For this review, use the dimensioned drawing (mm, ordinates from the lowest corner) and the shaded views. A direction names the side the tool comes from. Give positions to 0.01 mm unless a question says otherwise; leave off trailing zeros. Write each loop counter-clockwise with the first axis right and the second up, starting at its lowest first coordinate (ties: lowest second). Pieces come first, ordered by that corner, then holes. Notation, with made-up numbers: (8.25, 88) -> (61.25, 88) arc R28 cw to (61.25, 109) -> close; hole circle Ø1 at (3, -9.5). An arc over 180 degrees is marked (long way). Return JSON: item names as keys, results as strings.
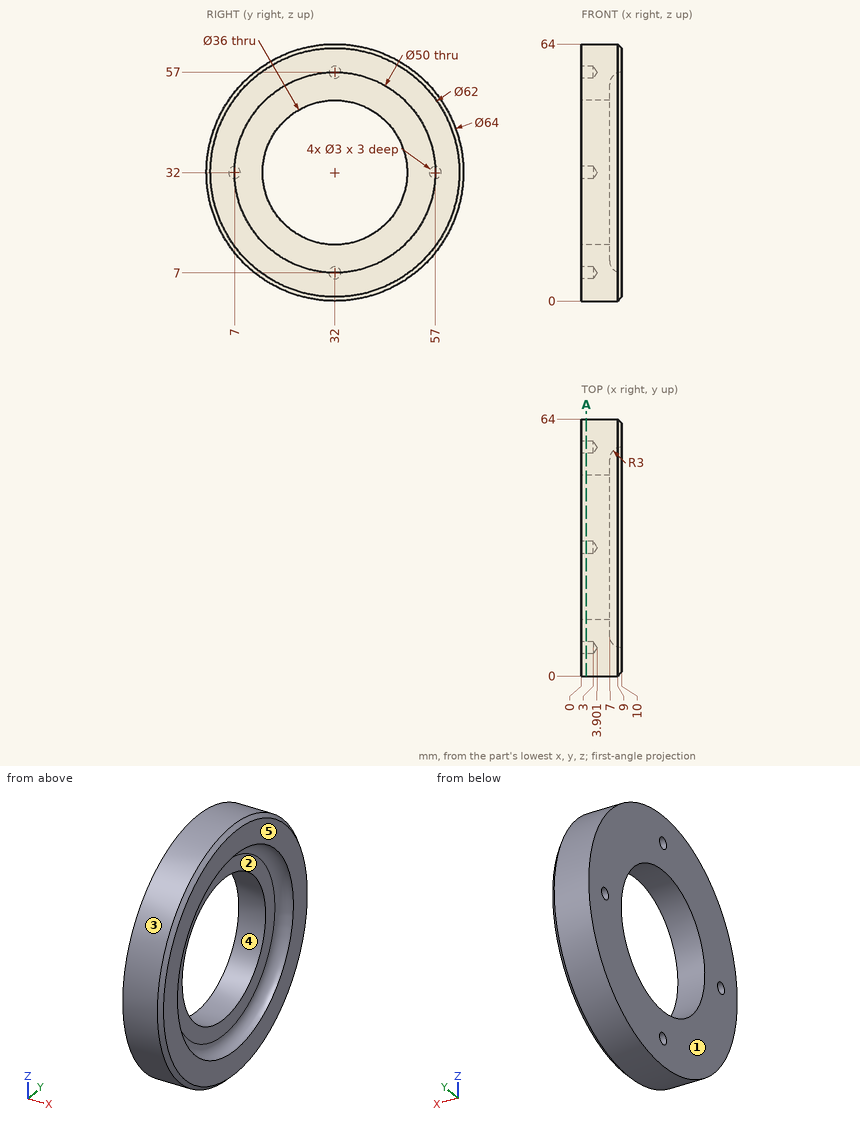
1. Add section A-A, the plane x = 1.25. State the section outline as (y, z) points, plus the area to 3 significant figures.
Results found:
{"outline": "circle Ø64 at (32, 32); hole circle Ø3 at (7, 32); hole circle Ø36 at (32, 32); hole circle Ø3 at (32, 7); hole circle Ø3 at (32, 57); hole circle Ø3 at (57, 32)", "area": "2,170 mm²"}
2. For the marked faces 1 and 2, list the 3-axis set-ups (+Z, -Z, +X, -X, +Y, -Y) from which the entire face can be reached by the end or side of a thin tool; tool diameter is ignored.
Results found:
{"face 1": "+Z, -Z, -X, +Y, -Y", "face 2": "+X"}
3. The part is to be moulded in two halves that separate along Z. For the marked faces 3, 4 and 5, say which applies: +Z half, -Z half, draft (parallel to the pull), parting line (faces both ways), or undercut.
Results found:
{"face 3": "parting line", "face 4": "undercut", "face 5": "draft"}
4. For pin 1 (5 mm diameter, centred on x = 4.5, y = 17, fed in from -Z); pin 2 (5 mm diameter, centred on x = 6.5, y = 38.5, fed in from +Z); pin 3 (3 mm diameter, centred on x = 5.5, z = 38, fed in from +Y); pin 4 (1.5 mm diameter, centred on y = 7.5, z = 7.5, fed in from -X), all flat-tipped, find the tip position at first contact; note any pin that passes through.
Results found:
{"pin 1": "stops at z = 2.54", "pin 2": "stops at z = 63.75", "pin 3": "stops at y = 63.68", "pin 4": "passes through"}
5. To check wall thickness, follow probe 1 along Z at (x, y) = (1.6, 32); probe 2 along Z at (x, y) = (3.25, 32) (1 decimal). State the ranges of each line that lie inside material, in increasing order.
Results found:
{"probe 1": "z = 0 to 5.5, 8.5 to 14, 50 to 55.5, 58.5 to 64", "probe 2": "z = 0 to 5.9, 8.1 to 14, 50 to 55.9, 58.1 to 64"}
